```python
from build123d import *

# Parameters (mm, degrees)
CLAMP_DEPTH      = 8
SKETCH2_R        = 2.1
SCREW_HOLE_DEPTH = 32.472209964


with BuildPart() as part:
    # Sketch1 → Clamp (new body)
    with BuildSketch(Plane.XY):
        with BuildLine():
            Line((-22.5, -7.5), (-13, -7.5))
            Line((-13, -7.5), (-13, 0))
            ThreePointArc((-13, 0), (0, 13), (13, 0))
            Line((13, 0), (13, -7.5))
            Line((13, -7.5), (22.5, -7.5))
            Line((22.5, -7.5), (22.5, -10.5))
            Line((22.5, -10.5), (10, -10.5))
            Line((10, -10.5), (10, 0))
            ThreePointArc((10, 0), (0, 10), (-10, 0))
            Line((-10, 0), (-10, -10.5))
            Line((-10, -10.5), (-22.5, -10.5))
            Line((-22.5, -10.5), (-22.5, -7.5))
        make_face()
    extrude(amount=CLAMP_DEPTH)

    # Sketch2 → Screw Hole (cut, through all)
    with BuildSketch(Plane(origin=(0, -7.5, 0), x_dir=(1, 0, 0), z_dir=(0, 1, 0))):
        with Locations(Location((-17.75, -4, 0), (0, 0, 270))):
            Circle(SKETCH2_R)
        with Locations(Location((17.75, -4, 0), (0, 0, 270))):
            Circle(SKETCH2_R)
    extrude(amount=-SCREW_HOLE_DEPTH, mode=Mode.SUBTRACT)


solid = part.part
```
Geometry: final body of the model. Coordinates: model frame, mm. A direction names the side the tool comes from. Round coordinates to 2 decimals unless told otherwise and drop trailing zeros. Order: outer loops, then holes, each group sorted by start corner. A loop starts at its lowest first (then second) coordinate and runs counter-clockwise, first axis right, second up. Notation, with made-up numbers: (0.25, 26) -> (46.25, 26) arc R31 cw to (46.25, 52) -> close; hole circle Ø6 at (45.25, 3). An arc over 180 degrees is marked (long way). Use one line per item in the form item = value.
(1) First-contact query: pin 1 Ø2 at (y, z) = (-2.5, 4.5) entering from -X; pin 2 Ø2 at (x, y) = (-15, -3) entering from -Z; pin 3 Ø4 at (y, z) = (1.5, 7) entering from +X. Flat tips, straight axial feed; report the tip coordinate or a pass-through.
Results list:
pin_1 = -13
pin_2 = through
pin_3 = 13
(2) Section B-B on x = -17.75. Return loops of the section in (y, z).
Results list:
outline = (-10.5, 0) -> (-7.5, 0) -> (-7.5, 1.9) -> (-10.5, 1.9) -> close; (-10.5, 6.1) -> (-7.5, 6.1) -> (-7.5, 8) -> (-10.5, 8) -> close
(3) Access query for faces 5 (the face through (19.52, -8.98, 5.13)), 6 (the face through (-13, -4, 4)), 7 (the face through (10, -5, 4)). Directions: +Z, -Z, +X, -X, +Y, -Y. A direction counts if a zero-diameter tool reaches every point of the face in a straight line with its end or side. Return the directions, or none.
Results list:
face_5 = +Y, -Y
face_6 = +Z, -Z, -X, +Y
face_7 = +Z, -Z, -Y
(4) Draft query along X for faces 1 (the face through (-10, -5, 4)), 2 (the face through (0, 10, 4)), 3 (the face through (13, -4, 4)), 4 (the face through (15.6, -7.5, 3.1)). Return one class per face: pulls with the +X half, pulls with the -X half, needs draft (parallel to the pull), parting line crosses it, or undercut.
Results list:
face_1 = undercut
face_2 = undercut
face_3 = pulls with the +X half
face_4 = needs draft
(5) Section D-D on z = 0.75. Return loops of the section in (x, y).
Results list:
outline = (-22.5, -10.5) -> (-10, -10.5) -> (-10, 0) arc R10 cw to (10, 0) -> (10, -10.5) -> (22.5, -10.5) -> (22.5, -7.5) -> (13, -7.5) -> (13, 0) arc R13 ccw to (-13, 0) -> (-13, -7.5) -> (-22.5, -7.5) -> close
(6) Ray query, probe 1 along X at (y, z) = (-8.85, 4); probe 2 along X at (y, z) = (-0.5, 7.5); probe 3 along X at (y, z) = (6.75, 6). Return the intervals inside material, ascending. Write a range as [from, to].
Results list:
probe_1 = [-22.5, -19.85], [-15.65, -10], [10, 15.65], [19.85, 22.5]
probe_2 = [-13, -10], [10, 13]
probe_3 = [-11.11, -7.38], [7.38, 11.11]
(7) Section C-C on z = 4. Return loops of the section in (x, y).
Results list:
outline = (-22.5, -10.5) -> (-19.85, -10.5) -> (-19.85, -7.5) -> (-22.5, -7.5) -> close; (-15.65, -10.5) -> (-10, -10.5) -> (-10, 0) arc R10 cw to (10, 0) -> (10, -10.5) -> (15.65, -10.5) -> (15.65, -7.5) -> (13, -7.5) -> (13, 0) arc R13 ccw to (-13, 0) -> (-13, -7.5) -> (-15.65, -7.5) -> close; (19.85, -10.5) -> (22.5, -10.5) -> (22.5, -7.5) -> (19.85, -7.5) -> close
(8) Section A-A on y = -1.75. Return loops of the section in (x, z), and give its area (3 significant figures).
Results list:
outline = (-13, 0) -> (-10, 0) -> (-10, 8) -> (-13, 8) -> close; (10, 0) -> (13, 0) -> (13, 8) -> (10, 8) -> close
area = 48.0 mm^2
